For this review, take the finished solid that the model builds, in its own axes (mm). A direction names the side the tool comes from. Round coordinates to 2 decimals unless told otherwise and drop trailing zeros. Order: outer loops, then holes, each group sorted by start corner. A loop starts at its lowest first (then second) coordinate and runs counter-clockwise, first axis right, second up. Notation, with made-up numbers: (44.25, 2) -> (77.25, 2) arc R26 cw to (77.25, 22) -> close; hole circle Ø1 at (7, 5). An arc over 180 degrees is marked (long way). Put each result on its own line as item: value. Start each with the question number.
```python
from build123d import *

# Parameters (mm, degrees)
SKETCH1_W            = 89
SKETCH1_H            = 5
BOSS_EXTRUDE1_DEPTH  = 10.14943
SKETCH2_W            = 85.527
SKETCH2_H            = 1.6
CUT_EXTRUDE1_DEPTH   = 7.7558
SKETCH3_W            = 117.05158
SKETCH3_H            = 1.6
BOSS_EXTRUDE2_DEPTH  = 15
M3_CLEARANCE_HOLE1_D = 3.6


with BuildPart() as part:
    # Sketch1 → Boss-Extrude1 (new body)
    with BuildSketch(Plane(origin=(0, 0, 0), x_dir=(1, 0, 0), z_dir=(0, 1, 0))):
        Rectangle(SKETCH1_W, SKETCH1_H)
    extrude(amount=BOSS_EXTRUDE1_DEPTH)

    # Sketch2 → Cut-Extrude1 (cut)
    with BuildSketch(Plane(origin=(0, 10.14943, 0), x_dir=(1, 0, 0), z_dir=(0, 1, 0))):
        with Locations((0.0912, -0.097552871)):
            Rectangle(SKETCH2_W, SKETCH2_H)
    extrude(amount=-CUT_EXTRUDE1_DEPTH, mode=Mode.SUBTRACT)

    # Sketch3 → Boss-Extrude2 (add)
    with BuildSketch(Plane.XZ):
        with Locations((-0.14221, 0.097552871)):
            Rectangle(SKETCH3_W, SKETCH3_H)
    extrude(amount=BOSS_EXTRUDE2_DEPTH)

    # M3 Clearance Hole1 (through all)
    with Locations(Plane.XY.offset(0.897552871)):
        with Locations((-54.14221, -5.5258), (53.85779, -5.5258)):
            Hole(M3_CLEARANCE_HOLE1_D / 2)


solid = part.part
```
Item 1: Consider section B-B, the plane x = -25. Write out the cut boundary in (y, z), plus the area to 3 significant figures.
Item 2: Insertion check: pin 1 Ø0.8 at (y, z) = (5, 0.5) entering from +X; pin 2 Ø0.5 at (x, z) = (3, 2) entering from -Y; pin 3 Ø2.5 at (y, z) = (6, 0.5) entering from -X. Each pin has a flat end and moves straight along its axis. Give the tip position at first contact, or say it passes through.
Item 3: Consider section A-A, the plane y = 6.25. Write out the cut boundary in (x, z), plus the area to 3 significant figures.
Item 4: Consider section C-C, the plane y = -12.5. Write out the cut boundary in (x, z), plus the area to 3 significant figures.
Item 5: Tool access review of faces 1 (the face through (-1, 6, -0.702)), 2 (the face through (-1, 0, -2)), 3 (the face through (-1, -7, 0.898)): name each direction out of +Z, -Z, +X, -X, +Y, -Y from which nothing blocks a thin tool from reaching the whole face with its end or side.
Item 6: For L1, parallel to Z at x = 25, y = 7.25; L2, parallel to Y at x = 1.5, z = -1.35; L3, parallel to X at y = 5.75, z = 1.25, list the stretches that pass through material, from the lowest coordinate up.
Item 7: Mouldability with a two-part tool opening along X and no side actions: class faces 4 (the face through (-44.5, 5, 0)), 5 (the face through (-1, 5, -2.5)), 6 (the face through (-52.344, -5.447, 0.086)), 7 (the face through (44.5, 5, 0)) as +X half, -X half, draft (parallel to the pull), parting line (faces both ways), or undercut.
Evaluation:
1. outline: (-15, -0.7) -> (0, -0.7) -> (0, -2.5) -> (10.15, -2.5) -> (10.15, -0.7) -> (2.39, -0.7) -> (2.39, 0.9) -> (10.15, 0.9) -> (10.15, 2.5) -> (0, 2.5) -> (0, 0.9) -> (-15, 0.9) -> close
1. area: 62.3 mm^2
2. pin 1: stops at x = 44.5
2. pin 2: stops at y = 0
2. pin 3: stops at x = -44.5
3. outline: (-44.5, -2.5) -> (44.5, -2.5) -> (44.5, 2.5) -> (-44.5, 2.5) -> close; hole (-42.67, -0.7) -> (42.85, -0.7) -> (42.85, 0.9) -> (-42.67, 0.9) -> close
3. area: 308 mm^2
4. outline: (-58.67, -0.7) -> (58.38, -0.7) -> (58.38, 0.9) -> (-58.67, 0.9) -> close
4. area: 187 mm^2
5. face 1: +Y
5. face 2: -Z, +X, -X, -Y
5. face 3: +Z, +X, -X, -Y
6. L1: z = -2.5 to -0.7, 0.9 to 2.5
6. L2: y = 0 to 10.15
6. L3: x = -44.5 to 44.5
7. face 4: -X half
7. face 5: draft
7. face 6: undercut
7. face 7: +X half
